from build123d import *

# Parameters (mm, degrees)
ESQUISSE2_W        = 18
ESQUISSE2_H        = 18
BOSS_EXTRU_1_DEPTH = 13.6
ESQUISSE3_W        = 2.8
ESQUISSE3_H        = 0.8
BOSS_EXTRU_2_DEPTH = 8.4


with BuildPart() as part:
    # Esquisse1 → Révolution1 (revolve)
    with BuildSketch(Plane.XY, mode=Mode.PRIVATE) as r_volution1_sk:
        with BuildLine():
            Line((0, 19), (0, 0))
            Line((0, 0), (0, -20))
            Line((0, -20), (8, -20))
            Line((8, -20), (8, 0))
            Line((8, 0), (10, 0))
            Line((10, 0), (10, 9))
            Line((10, 9), (7, 9))
            Line((7, 9), (7, 15))
            Line((7, 15), (12, 15))
            Line((12, 15), (12, 17.5))
            ThreePointArc((12, 17.5), (6.046693311, 18.62354649), (0, 19))
        make_face()
    revolve(r_volution1_sk.sketch.rotate(Axis((0, 19, 0), (0, 1, 0)), 90), axis=Axis((0, 19, 0), (0, 1, 0)))

    # Esquisse2 → Boss.-Extru.1 (add)
    with BuildSketch(Plane.XZ.offset(20)):
        Rectangle(ESQUISSE2_W, ESQUISSE2_H)
    extrude(amount=BOSS_EXTRU_1_DEPTH)

    # Esquisse3 → Boss.-Extru.2 (add)
    with BuildSketch(Plane.XZ.offset(33.6)):
        with Locations((-6, 7.65)):
            Rectangle(ESQUISSE3_W, ESQUISSE3_H)
        with Locations((6, 7.65)):
            Rectangle(ESQUISSE3_W, ESQUISSE3_H)
        with Locations((6, -7.65)):
            Rectangle(ESQUISSE3_W, ESQUISSE3_H)
        with Locations((-6, -7.65)):
            Rectangle(ESQUISSE3_W, ESQUISSE3_H)
    extrude(amount=BOSS_EXTRU_2_DEPTH)


solid = part.part
The model under review builds one solid part; all positions refer to its coordinate system, in mm. A direction names the side the tool comes from. Coordinates: 2 decimals unless noted, no trailing zeros. Write each loop counter-clockwise with the first axis right and the second up, starting at its lowest first coordinate (ties: lowest second). Pieces come first, ordered by that corner, then holes. Notation, with made-up numbers: (17, -0.75) -> (45, -0.75) arc R25 ccw to (45, 16.25) -> close; hole circle Ø8 at (-10.5, 88). An arc over 180 degrees is marked (long way). Answer in a Markdown table with one row per item.
1. We need section D-D, the plane x = 6. State the section outline as (y, z) points.
Answers below:
| item | result |
|---|---|
| outline | (-42, -8.05) -> (-33.6, -8.05) -> (-33.6, -9) -> (-20, -9) -> (-20, -5.29) -> (0, -5.29) -> (0, -8) -> (9, -8) -> (9, -3.61) -> (15, -3.61) -> (15, -10.39) -> (17.5, -10.39) arc R48.38 ccw to (17.5, 10.39) -> (15, 10.39) -> (15, 3.61) -> (9, 3.61) -> (9, 8) -> (0, 8) -> (0, 5.29) -> (-20, 5.29) -> (-20, 9) -> (-33.6, 9) -> (-33.6, 8.05) -> (-42, 8.05) -> (-42, 7.25) -> (-33.6, 7.25) -> (-33.6, -7.25) -> (-42, -7.25) -> close |
2. We need section C-C, the plane y = 5.5. State the section outline as (x, z) points.
Answers below:
| item | result |
|---|---|
| outline | circle Ø20 at (0, 0) |
3. We need section A-A, the plane x = 0. State the section outline as (y, z) points, and give its area (3 significant figures).
Answers below:
| item | result |
|---|---|
| outline | (-33.6, -9) -> (-20, -9) -> (-20, -8) -> (0, -8) -> (0, -10) -> (9, -10) -> (9, -7) -> (15, -7) -> (15, -12) -> (17.5, -12) arc R48.75 ccw to (17.5, 12) -> (15, 12) -> (15, 7) -> (9, 7) -> (9, 10) -> (0, 10) -> (0, 8) -> (-20, 8) -> (-20, 9) -> (-33.6, 9) -> close |
| area | 913 mm^2 |
4. For faces 1 (the flat face through (0, -27, -9)), 2 (the flat face through (-8, -20, 2)), 3 (the flat face through (0, -27, 9)), 4 (the flat face through (-6, -38, 7.25)), list the 3-axis set-ups (+Z, -Z, +X, -X, +Y, -Y) from which the entire face can be reached by the end or side of a thin tool; tool diameter is ignored.
Answers below:
| item | result |
|---|---|
| face 1 | -Z, +X, -X, -Y |
| face 2 | none |
| face 3 | +Z, +X, -X, -Y |
| face 4 | +X, -X, -Y |
5. Clearance check with flat-ended pins moving along their axes: pin 1 Ø10 at (y, z) = (-33, 5) entering from +X; pin 2 Ø0.8 at (x, y) = (6.5, -37) entering from -Z; pin 3 Ø6 at (x, y) = (9, 0.5) entering from +Z. State where each tip first meets the part, or that it passes through.
Answers below:
| item | result |
|---|---|
| pin 1 | stops at x = 9 |
| pin 2 | stops at z = -8.05 |
| pin 3 | stops at z = 8 |
6. We need section B-B, the plane z = 0. State the section outline as (x, y) points, and give its area (3 significant figures).
Answers below:
| item | result |
|---|---|
| outline | (-12, 15) -> (-7, 15) -> (-7, 9) -> (-10, 9) -> (-10, 0) -> (-8, 0) -> (-8, -20) -> (-9, -20) -> (-9, -33.6) -> (9, -33.6) -> (9, -20) -> (8, -20) -> (8, 0) -> (10, 0) -> (10, 9) -> (7, 9) -> (7, 15) -> (12, 15) -> (12, 17.5) arc R48.75 ccw to (-12, 17.5) -> close |
| area | 913 mm^2 |
7. Wall thickness on probe 1 along Y at (x, z) = (-0.5, 8.25); probe 2 along Y at (x, z) = (6, -7); probe 3 along X at (y, z) = (-24.5, 2.75): over which ranges is each line inside the solid? List them lowest first. Write a range as [from, to].
Answers below:
| item | result |
|---|---|
| probe 1 | y = [-33.6, -20], [0, 9], [15, 18.29] |
| probe 2 | y = [-33.6, -20], [0, 9], [15, 18.12] |
| probe 3 | x = [-9, 9] |
8. Draft analysis for pull direction Z (two halves, no side actions). For faces 5 (the flat face through (-7, 9, -2)), 6 (the flat face through (-6, -38, -8.05)), 7 (the flat face through (0, -33.6, 0)), state which applies: +Z half, -Z half, draft (parallel to the pull), parting line (faces both ways), or undercut.
Answers below:
| item | result |
|---|---|
| face 5 | draft |
| face 6 | -Z half |
| face 7 | undercut |
